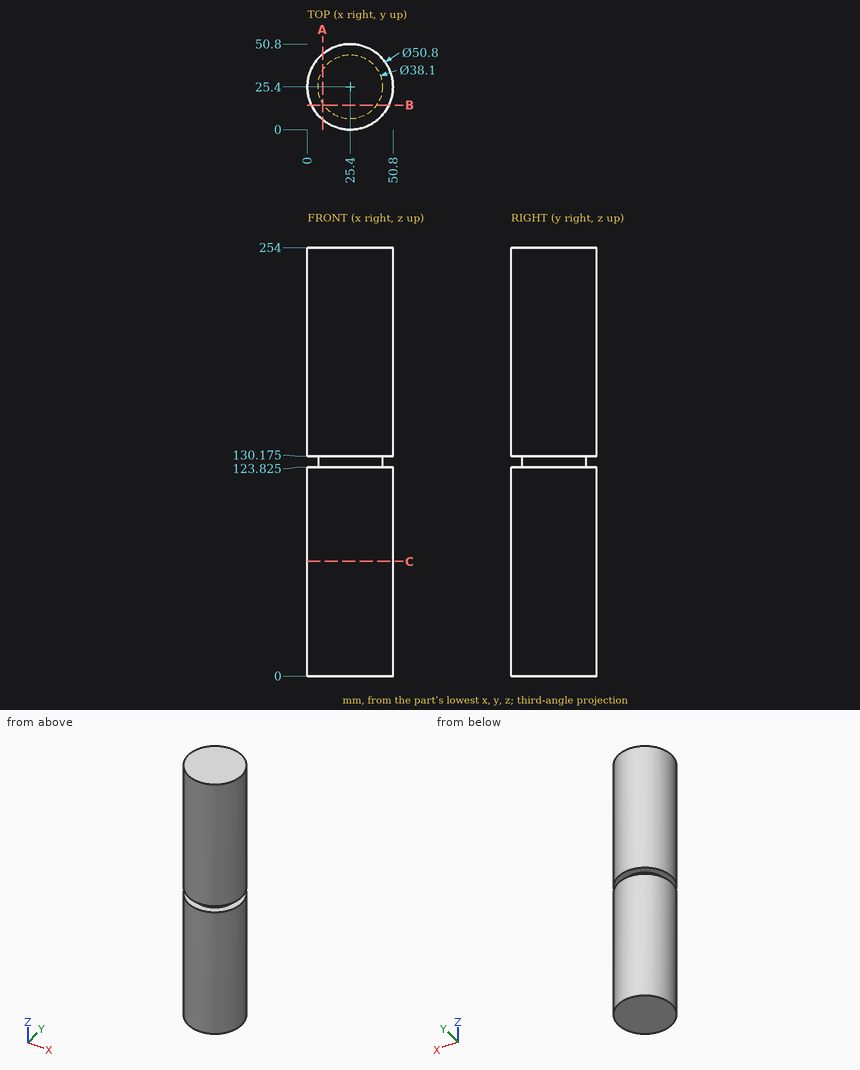
Can you work these out from the drawing? Everything is in mm from the part's minimum corner. Give positions to 0.01 mm unless a question says otherwise; leave off trailing zeros. Loops run counter-clockwise (first coordinate to the right, second up) from the corner with the lowest first, then second, coordinate; pieces in that order, holes last. Notation, with made-up numbers: (-39.75, 17) - (9.25, 17) arc R14 ccw to (9.25, 28) - close; hole circle Ø9 at (54, -4). An arc over 180 degrees is marked (long way). Answer as a JSON object with one key per item and string values.
Q1. Imagine slicing it at A-A on x = 9. Write out the boundary of the cut face in (y, z) (3 decimals), plus the area to 3 significant figures.
Geometry says:
{"outline": "(6.004, 0) - (44.796, 0) - (44.796, 123.825) - (35.092, 123.825) - (35.092, 130.175) - (44.796, 130.175) - (44.796, 254) - (6.004, 254) - (6.004, 130.175) - (15.708, 130.175) - (15.708, 123.825) - (6.004, 123.825) - close", "area": "9,730 mm²"}
Q2. Imagine slicing it at B-B on y = 14.5. Write out the boundary of the cut face in (x, z) (3 decimals), plus the area to 3 significant figures.
Geometry says:
{"outline": "(2.458, 0) - (48.342, 0) - (48.342, 123.825) - (41.023, 123.825) - (41.023, 130.175) - (48.342, 130.175) - (48.342, 254) - (2.458, 254) - (2.458, 130.175) - (9.777, 130.175) - (9.777, 123.825) - (2.458, 123.825) - close", "area": "11,600 mm²"}
Q3. Imagine slicing it at C-C on z = 68. Write out the boundary of the cut face in (x, y).
Geometry says:
{"outline": "circle Ø50.8 at (25.4, 25.4)"}
Q4. If I drill on L1, parallel to Z at x = 16, y = 7 (3 decimals); L2, parallel to Y at x = 25, z = 154.5; L3, parallel to X at y = 13, z = 34, over which ranges is the centre line in solid material (lowest first)?
Geometry says:
{"L1": "0 to 123.825, 130.175 to 254", "L2": "0 to 50.8", "L3": "3.23 to 47.57"}
Q5. Will these pins go through, and if not, where does the flat tip stop? P1, Ø3, axis at y = 43, z = 221.5, coming from the +X side; P2, Ø8, axis at x = 43.5, z = 117, coming from the -Y side; P3, Ø10, axis at x = 20, z = 175, coming from the +Y side.
Geometry says:
{"P1": "x = 45.05", "P2": "y = 4.27", "P3": "y = 50.8"}
